```python
from build123d import *

# Parameters (mm, degrees)
SKETCH1_W           = 254
SKETCH1_H           = 114.3
BOSS_EXTRUDE1_DEPTH = 63.5
CHAMFER1_SIZE       = 5.08
SKETCH4_W           = 25
SKETCH4_H           = 58
CUT_EXTRUDE2_DEPTH  = 11.189999972
SHELL3_T            = -2.54
SKETCH6_W           = 30.08
SKETCH6_H           = 63.08
BOSS_EXTRUDE2_DEPTH = 12.7
SKETCH5_W           = 20
SKETCH5_H           = 40
CUT_EXTRUDE5_DEPTH  = 53.310000028
SKETCH7_R           = 4.85
CUT_EXTRUDE6_DEPTH  = 25.4
SKETCH8_R           = 2.2
CUT_EXTRUDE7_DEPTH  = 53.310000028
CUT_EXTRUDE9_START  = -127
CUT_EXTRUDE9_DEPTH  = 38.1
CUT_EXTRUDE10_DEPTH = 64.5
SKETCH12_W          = 56
SKETCH12_H          = 18
CUT_EXTRUDE12_DEPTH = 2.54


with BuildPart() as part:
    # Sketch1 → Boss-Extrude1 (new body)
    with BuildSketch(Plane(origin=(0, 0, 0), x_dir=(1, 0, 0), z_dir=(0, 1, 0))):
        with Locations((-127, 57.15)):
            Rectangle(SKETCH1_W, SKETCH1_H)
    extrude(amount=BOSS_EXTRUDE1_DEPTH)

    # Chamfer1
    chamfer1_edges = [part.edges().sort_by_distance(p)[0] for p in [
        (-254, 63.5, -57.15),
        (-127, 63.5, 0),
        (0, 63.5, -57.15),
        (0, 31.75, 0),
        (-254, 31.75, 0),
        (-254, 31.75, -114.3),
        (0, 31.75, -114.3),
        (-127, 63.5, -114.3),
    ]]
    chamfer(chamfer1_edges, length=CHAMFER1_SIZE)

    # Sketch4 → Cut-Extrude2 (cut)
    with BuildSketch(Plane(origin=(0, 63.5, 0), x_dir=(1, 0, 0), z_dir=(0, 1, 0))):
        with Locations((-198.12, 47.15)):
            Rectangle(SKETCH4_W, SKETCH4_H)
    extrude(amount=-CUT_EXTRUDE2_DEPTH, mode=Mode.SUBTRACT)

    # Shell3
    shell3_openings = [part.faces().sort_by_distance(p)[0] for p in [
        (-127, 0, -57.15),
    ]]
    offset(amount=SHELL3_T, openings=shell3_openings, kind=Kind.INTERSECTION)

    # Sketch6 → Boss-Extrude2 (add)
    with BuildSketch(Plane.XZ.offset(-49.770000028)):
        with Locations((-198.12, -47.15)):
            Rectangle(SKETCH6_W, SKETCH6_H)
    extrude(amount=BOSS_EXTRUDE2_DEPTH)

    # Sketch5 → Cut-Extrude5 (cut, through all)
    with BuildSketch(Plane(origin=(0, 52.310000028, 0), x_dir=(1, 0, 0), z_dir=(0, 1, 0))):
        with Locations((-198.12, 47.15)):
            Rectangle(SKETCH5_W, SKETCH5_H)
    extrude(amount=-CUT_EXTRUDE5_DEPTH, mode=Mode.SUBTRACT)

    # Sketch7 → Cut-Extrude6 (cut)
    with BuildSketch(Plane.XY):
        with Locations((-63.5, 25.4)):
            Circle(SKETCH7_R)
    extrude(amount=-CUT_EXTRUDE6_DEPTH, mode=Mode.SUBTRACT)

    # Sketch8 → Cut-Extrude7 (cut, through all)
    with BuildSketch(Plane(origin=(0, 52.310000028, 0), x_dir=(1, 0, 0), z_dir=(0, 1, 0))):
        with Locations((-203.12, 71.9)):
            Circle(SKETCH8_R)
        with Locations((-193.12, 71.9)):
            Circle(SKETCH8_R)
        with Locations((-193.12, 22.4)):
            Circle(SKETCH8_R)
        with Locations((-203.12, 22.4)):
            Circle(SKETCH8_R)
    extrude(amount=-CUT_EXTRUDE7_DEPTH, mode=Mode.SUBTRACT)

    # Sketch9 → Cut-Extrude9 (cut, symmetric)
    with BuildSketch(Plane(origin=(0, 0, 0), x_dir=(0, 0, -1), z_dir=(1, 0, 0)).offset(CUT_EXTRUDE9_START)):
        Polygon((2.54, 0), (3.81, 0), (3.81, 3.81), (1.27, 3.81), (2.54, 1.27), align=None)
    cut_extrude9 = extrude(amount=CUT_EXTRUDE9_DEPTH, both=True, mode=Mode.SUBTRACT)

    # Mirror1: Cut-Extrude9 across plane
    add(cut_extrude9.mirror(Plane.XY.offset(-57.15)), mode=Mode.SUBTRACT)

    # Sketch10 → Cut-Extrude10 (cut, through all)
    with BuildSketch(Plane(origin=(0, 63.5, 0), x_dir=(1, 0, 0), z_dir=(0, 1, 0))):
        with BuildLine():
            ThreePointArc((-226.45590841, 77.22804441), (-237.729116487, 50.012112577), (-226.45590841, 22.796180745))
            ThreePointArc((-226.45590841, 22.796180745), (-216.854647797, 22.796180745), (-216.854647797, 32.397441358))
            ThreePointArc((-216.854647797, 32.397441358), (-224.150883513, 50.012112577), (-216.854647797, 67.626783797))
            ThreePointArc((-216.854647797, 67.626783797), (-216.854647797, 77.22804441), (-226.45590841, 77.22804441))
        make_face()
    extrude(amount=-CUT_EXTRUDE10_DEPTH, mode=Mode.SUBTRACT)

    # Sketch12 → Cut-Extrude12 (cut)
    with BuildSketch(Plane(origin=(0, 0, 0), x_dir=(0, 0, -1), z_dir=(1, 0, 0))):
        with Locations((57.15, 21.7)):
            Rectangle(SKETCH12_W, SKETCH12_H)
    extrude(amount=-CUT_EXTRUDE12_DEPTH, mode=Mode.SUBTRACT)


solid = part.part
```
Build history of the part. All positions in model axes, mm. A direction names the side the tool comes from. Round coordinates to 2 decimals unless told otherwise and drop trailing zeros. Write each loop counter-clockwise with the first axis right and the second up, starting at its lowest first coordinate (ties: lowest second). Pieces come first, ordered by that corner, then holes. Notation, with made-up numbers: (47, -10.5) - (76, -10.5) arc R15 ccw to (76, -1.5) - close; hole circle Ø10 at (4.25, 35.25). An arc over 180 degrees is marked (long way). Write each question's results on one line, items separated by ' | '. Start each with the question number.
Item 1: Drop flat-ended pins along their axis: P1, Ø1, axis at x = -185, z = -15, coming from the -Y side; P2, Ø3.5, axis at x = -193.12, z = -22.4, coming from the -Y side; P3, Ø2, axis at x = -1.5, y = 20, coming from the +Z side; P4, Ø1.4, axis at y = 2, z = -112.5, coming from the -X side. Give the stop position or say it passes through.
Item 2: Saw through at B-B (z = -37). State how many separate pieces and enclosed holes the cut face has, and give its area (3 significant figures).
Item 3: Which spindle directions (+Z, -Z, +X, -X, +Y, -Y) get a long thin tool onto all of the face, cutting with end or side? Do faces 5 (the face through (-185.62, 58, -47)), 6 (the face through (-198, 45, -27.15)), 7 (the face through (-213.16, 49, -48)). Say none if no direction does.
Item 4: Saw through at A-A (x = -63.5). Write the cut outline in (y, z).
Item 5: Wall check: L1, parallel to X at y = 43.25, z = -22.4; L2, parallel to Z at x = -193, y = 46; L3, parallel to X at y = 42, z = -22. Give the ranges that are in metal, low to high. Write a range as [from, to].
Item 6: Mould opens along Y. For faces 1 (the face through (-2.58, 61, -56.42)), 2 (the face through (0, 35, -56)), 3 (the face through (-208.4, 37.07, -46.7)), 4 (the face through (-68.345, 25.613, -1.252)) say: pulls with the +Y half, pulls with the -Y half, needs draft (parallel to the pull), parting line crosses it, or undercut.
Item 7: Saw through at D-D (z = -94). Write the cut outline in (x, y).
Item 8: Saw through at C-C (x = -152). Write the cut outline in (y, z).
Results are:
1) P1: stops at y = 60.96 | P2: passes through | P3: stops at z = -2.58 | P4: stops at x = -251.42
2) separate pieces: 4 | enclosed holes: 0 | area: 992 mm²
3) face 5: +Y | face 6: +Y, -Y | face 7: -Y
4) outline: (0, -114.3) - (58.42, -114.3) - (63.5, -109.22) - (63.5, -5.08) - (58.42, 0) - (30.25, 0) - (30.25, -2.54) - (57.37, -2.54) - (60.96, -6.13) - (60.96, -108.17) - (57.37, -111.76) - (0, -111.76) - close; (0, -2.54) - (20.55, -2.54) - (20.55, 0) - (0, 0) - close
5) L1: x = [-254, -251.46], [-213.16, -205.32], [-200.92, -195.32], [-190.92, -183.08], [-2.54, 0] | L2: z = [-114.3, -111.76], [-78.69, -74.1], [-69.7, -67.15], [-27.15, -24.6], [-20.2, -15.61], [-2.54, 0] | L3: x = [-254, -251.46], [-213.16, -205.28], [-200.96, -195.28], [-190.96, -183.08], [-2.54, 0]
6) face 1: pulls with the +Y half | face 2: needs draft | face 3: pulls with the -Y half | face 4: undercut
7) outline: (-254, 0) - (-251.46, 0) - (-251.46, 57.37) - (-247.87, 60.96) - (-6.13, 60.96) - (-2.54, 57.37) - (-2.54, 0) - (0, 0) - (0, 58.42) - (-5.08, 63.5) - (-248.92, 63.5) - (-254, 58.42) - close
8) outline: (0, -114.3) - (58.42, -114.3) - (63.5, -109.22) - (63.5, -5.08) - (58.42, 0) - (0, 0) - (0, -2.54) - (1.27, -2.54) - (3.81, -1.27) - (3.81, -2.54) - (57.37, -2.54) - (60.96, -6.13) - (60.96, -108.17) - (57.37, -111.76) - (3.81, -111.76) - (3.81, -113.03) - (1.27, -111.76) - (0, -111.76) - close
